Here's how the part is built. I have some questions about the finished solid (model axes, mm). A direction names the side the tool comes from. Coordinates: 2 decimals unless noted, no trailing zeros. Order: outer loops, then holes, each group sorted by start corner. A loop starts at its lowest first (then second) coordinate and runs counter-clockwise, first axis right, second up. Notation, with made-up numbers: (-30.5, 84) - (-5.5, 84) arc R24 cw to (-5.5, 102) - close; hole circle Ø4 at (19, 13.25). An arc over 180 degrees is marked (long way). Use one line per item in the form item = value. Start each with the question number.
from build123d import *

# Parameters (mm, degrees)
FILLET3_R = 1.7
FILLET4_R = 1.7


with BuildPart() as part:
    # Sketch1 → Revolve2 (revolve)
    with BuildSketch(Plane.XY):
        Polygon((-71.835738672, 25.657855278), (-71.835738672, 31.241430002), (-90.666618133, 31.241430002), (-90.666618133, 40.656869732), (-66.142682091, 40.656869732), (-66.142682091, 31.241430002), (-58.588433936, 31.241430002), (-58.588433936, 40.656869732), (-54.866050787, 40.656869732), (-54.866050787, 25.657855278), (-66.142682091, 25.657855278), (-66.142682091, 19.964798697), (-69.974547098, 19.964798697), (-69.974547098, 25.657855278), align=None)
    revolve(axis=Axis((-23.866050787, 40.656869732, 0), (0, -1, 0)))

    # Fillet3
    fillet3_edges = [part.edges().sort_by_distance(p)[0] for p in [
        (42.93451656, 40.656869732, 0),
    ]]
    fillet(fillet3_edges, radius=FILLET3_R)

    # Fillet4
    fillet4_edges = [part.edges().sort_by_distance(p)[0] for p in [
        (18.410580518, 25.657855278, 0),
    ]]
    fillet(fillet4_edges, radius=FILLET4_R)


solid = part.part
1) If we mould it in two halves opening along Z, with no side actions, what happens to faces 4 (the cylindrical face through (-19.83, 33.052, -30.736)), 5 (the flat face through (-10.8, 40.657, -28.5)), 6 (the cylindrical face through (-56.985, 36.015, -10.43)), 7 (the cylindrical face through (-13.47, 28.49, 46.83))? For each: pulls with the +Z half, pulls with the -Z half, needs draft (parallel to the pull), parting line crosses it, or undercut.
2) I need wall thicknesses on probe 1 along X at (y, z) = (34.25, 0); probe 2 along X at (y, z) = (32, 15); probe 3 along Z at (x, y) = (-26.5, 36.25). Which ranges of each line are inside material? Lowest first, please. Write a range as [from, to].
3) Suppose I cut it at B-B, the plane y = 34.75. List the corners of the cut face in (x, z) for me.
4) For pin 1 (1.5 mm diameter, centred on x = 18, y = 34, fed in from +Z); pin 2 (4 mm diameter, centred on y = 35, z = -38, fed in from +X); pin 3 (2 mm diameter, centred on y = 35, z = -14, fed in from +X); pin 4 (1 mm diameter, centred on x = -67.5, z = 52, fed in from -Y) (3 decimals), each with a flat end and sliding along its axis, tell me the tip position at first contact or that it passes through.
5) Which directions (+Z, -Z, +X, -X, +Y, -Y) give clear straight access to the entire face, cutting with the end or side of a thin tool? Please do faces 1 (the cylindrical face through (-9.38, 35.15, 65.21)), 2 (the flat face through (-21, 31.241, -35)), 3 (the flat face through (-49, 25.658, -39)).
From the geometry:
q1.face_4 = undercut
q1.face_5 = needs draft
q1.face_6 = undercut
q1.face_7 = parting line crosses it
q2.probe_1 = [-90.67, -66.14], [-58.59, -54.87], [7.13, 10.86], [18.41, 42.93]
q2.probe_2 = [-88.96, -63.39], [-55.18, -51], [3.26, 7.45], [15.66, 41.23]
q2.probe_3 = [-66.75, -42.19], [-34.62, -30.89], [30.89, 34.62], [42.19, 66.75]
q3.outline = circle Ø133.6 at (-23.87, 0); circle Ø69.44 at (-23.87, 0); hole circle Ø84.55 at (-23.87, 0); hole circle Ø62 at (-23.87, 0)
q4.pin_1 = 52.65
q4.pin_2 = 32.4
q4.pin_3 = 41.66
q4.pin_4 = through
q5.face_1 = +Y, -Y
q5.face_2 = +Y
q5.face_3 = -Y
